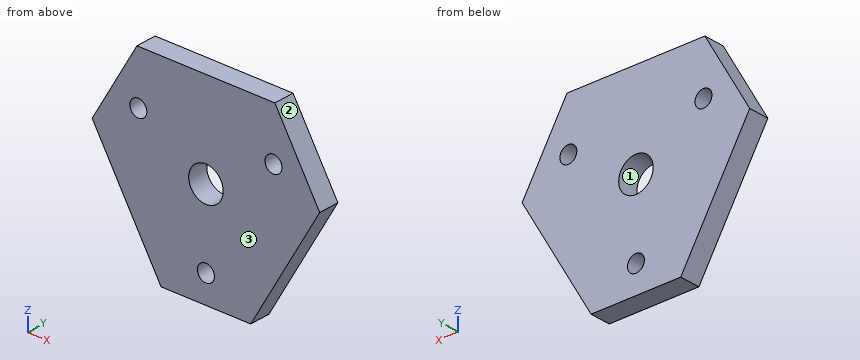
Autodesk Inventor part; units mm, degrees
ref_plane "YZ Plane" through (0, 0, 0) normal (1, 0, 0) x (0, 1, 0)
ref_plane "XZ Plane" through (0, 0, 0) normal (0, 1, 0) x (-1, 0, 0)
ref_plane "XY Plane" through (0, 0, 0) normal (0, 0, 1) x (1, 0, 0)
sketch "Skizze1" plane through (0, 0, 0) normal (0, 1, 0) x (-1, 0, 0)
  line L0 (0, 0) -> (46, 79.6743)
  line L1 (46, 79.6743) -> (-46, 79.6743)
  line L2 (-46, 79.6743) -> (0, 0)
  line L3 (0, 0) -> (0, 79.6743) construction
  line L4 (-46, 79.6743) -> (23, 39.8372) construction
  line L5 (46, 79.6743) -> (-23, 39.8372) construction
  dimension "d0" = 92
extrude "Extrusion1" add sketch "Skizze1" along normal mid plane 6
sketch "Skizze2" plane through (0, -3, 0) normal (0, -1, 0) x (1, 0, 0)
  line L0 (46, 79.6743) -> (-46, 79.6743)
  line L1 (-46, 79.6743) -> (0, 0)
  line L2 (0, 0) -> (46, 79.6743)
  line L3 (0, 0) -> (0, 0) construction
  line L4 (0, 0) -> (0, 79.6743) construction
  line L5 (-46, 79.6743) -> (0, 0)
  line L6 (46, 79.6743) -> (-46, 79.6743)
  line L7 (-23, 39.8372) -> (46, 79.6743) construction
  line L8 (23, 39.8372) -> (-46, 79.6743) construction
  line L9 (-33, 57.1577) -> (-20, 79.6743)
  point P0 (-33, 57.1577)
  point P1 (-20, 79.6743)
  point P2 (-26.5, 68.416)
  dimension "d31" = 26
extrude "Extrusion6" cut sketch "Skizze2" against normal blind 10 contours L9 L1 L0
mirror "Spiegeln1" about plane through (0, 0, 0) normal (1, 0, 0) of "Extrusion6"
sketch "Skizze7" plane through (0, -3, 0) normal (0, -1, 0) x (1, 0, 0)
  line L0 (0, 0) -> (-33, 57.1577)
  line L1 (-13, 22.5167) -> (13, 22.5167)
  line L2 (33, 57.1577) -> (0, 0)
  dimension "d38" = 26
extrude "Extrusion7" cut sketch "Skizze7" against normal blind 10
sketch "Skizze3" plane through (0, -3, 0) normal (0, -1, 0) x (1, 0, 0)
  line L0 (46, 79.6743) -> (-46, 79.6743)
  line L1 (-13, 22.5167) -> (13, 22.5167)
  line L2 (-20, 79.6743) -> (-33, 57.1577)
  line L3 (33, 57.1577) -> (20, 79.6743)
  point P0 (0, 0)
  point P1 (-19.5959, 64.3743)
  point P2 (19.5959, 64.3743)
  point P3 (0, 30.5167)
  point P4 (33.8756, 72.6743)
  point P5 (-26.5, 68.416)
  dimension "d41" = 8
  dimension "d42" = 8
  dimension "d43" = 8
  dimension "d44" = 15.3
hole "Bohrung1" at (-19.5959, -3, 64.3743) at (19.5959, -3, 64.3743) at (0, -3, 30.5167) direction (0, 1, 0) diameter 4.917 depth 6
sketch "Skizze8" plane through (0, -3, 0) normal (0, -1, 0) x (1, 0, 0)
  circle A0 centre (0, 52.5167) radius 5
  line L0 (-13, 22.5167) -> (13, 22.5167)
  point P0 (0, 0)
  point P1 (0, 22.5167)
  dimension "d45" = 30
  dimension "d46" = 10
extrude "Extrusion8" cut sketch "Skizze8" against normal blind 10
equation "\"d9\" = d8"
properties part number "Plate" material "Aluminium 6061"
Here's how the part is built. I have some questions about the finished solid (model axes, mm). Face numbers are marked on the shaded views. Coordinates: 2 decimals unless noted, no trailing zeros. Order: outer loops, then holes, each group sorted by start corner. A loop starts at its lowest first (then second) coordinate and runs counter-clockwise, first axis right, second up. Notation, with made-up numbers: M 74,-23.75 L 82,-23.75 A12 ccw 82,-19.75 Z; hole C 35,-8 d2. An arc over 180 degrees is marked long. Answer as CSV lines item,"result".
Item 1: We'd pull the mould along X, two halves only. Please class the marked faces 1, 2 and 3: +X half, -X half, draft (parallel to the pull), parting line (faces both ways), or undercut.
Results found:
face 1,"undercut"
face 2,"+X half"
face 3,"draft"
Item 2: If I drill on line 1 (Z direction, x = 0, y = 0.75); line 2 (X direction, y = 2.1, z = 64); line 3 (Z direction, x = 21.5, y = 1.55), over which ranges is the centre line in solid material (lowest first)?
Results found:
line 1,"22.52 to 28.06, 32.98 to 47.52, 57.52 to 79.67"
line 2,"-29.05 to -22.03, -17.17 to 17.17, 22.03 to 29.05"
line 3,"37.24 to 62.82, 65.93 to 77.08"
Item 3: Imagine slicing it at C-C on y = 2.15. Write out the boundary of the cut face in (x, z).
Results found:
outline,"M -33,57.16 L -13,22.52 L 13,22.52 L 33,57.16 L 20,79.67 L -20,79.67 Z; hole C -19.6,64.37 d4.92; hole C 0,52.52 d10; hole C 0,30.52 d4.92; hole C 19.6,64.37 d4.92"
Item 4: For pin 1 (4.5 mm diameter, centred on x = 19.6, z = 64.37, fed in from +Y), with a flat end and sliding along its axis, tell me the tip position at first contact or that it passes through.
Results found:
pin 1,"through"
Item 5: Imagine slicing it at B-B on z = 64. Write out the boundary of the cut face in (x, y), plus the area to 3 significant figures.
Results found:
outline,"M -29.05,-3 L -22.03,-3 L -22.03,3 L -29.05,3 Z; M -17.17,-3 L 17.17,-3 L 17.17,3 L -17.17,3 Z; M 22.03,-3 L 29.05,-3 L 29.05,3 L 22.03,3 Z"
area,"290 mm2"
Item 6: Imagine slicing it at A-A on x = 0. Write out the boundary of the cut face in (y, z), plus the area to 3 significant figures.
Results found:
outline,"M -3,22.52 L 3,22.52 L 3,28.06 L -3,28.06 Z; M -3,32.98 L 3,32.98 L 3,47.52 L -3,47.52 Z; M -3,57.52 L 3,57.52 L 3,79.67 L -3,79.67 Z"
area,"253 mm2"
Item 7: Imagine slicing it at D-D on z = 36.5. Write out the boundary of the cut face in (x, y).
Results found:
outline,"M -21.07,-3 L 21.07,-3 L 21.07,3 L -21.07,3 Z"
